from build123d import *

# Parameters (mm, degrees)
F1_DEPTH = 70
F2_R     = 50
F3_T     = -5


with BuildPart() as f1:
    # F0 (on Front) → F1 (new body)
    with BuildSketch(Plane.XZ):
        with BuildLine():
            Line((195.61244, 127.258498), (-44.38756, 127.258498))
            ThreePointArc((-44.38756, 127.258498), (-83.278433, 111.149371), (-99.38756, 72.258498))
            ThreePointArc((-99.38756, 72.258498), (-83.278433, 33.367625), (-44.38756, 17.258498))
            Line((-44.38756, 17.258498), (195.61244, 17.258498))
            ThreePointArc((195.61244, 17.258498), (234.503313, 33.367625), (250.61244, 72.258498))
            ThreePointArc((250.61244, 72.258498), (234.503313, 111.149371), (195.61244, 127.258498))
        make_face()
    extrude(amount=F1_DEPTH)

    # F2
    f2_edges = [f1.edges().sort_by_distance(p)[0] for p in [
        (75.61244, -70, 127.258498),
        (-99.38756, -70, 72.258498),
        (75.61244, -70, 17.258498),
        (250.61244, -70, 72.258498),
    ]]
    fillet(f2_edges, radius=F2_R)

    # F3
    f3_openings = [f1.faces().sort_by_distance(p)[0] for p in [
        (75.61244, 0, 72.258498),
    ]]
    offset(amount=F3_T, openings=f3_openings)


solid = f1.part
Geometry check sheet. Reference: the model listing, model coordinates, mm. A direction names the side the tool comes from. Give positions to 0.01 mm unless a question says otherwise; leave off trailing zeros. Loops run counter-clockwise (first coordinate to the right, second up) from the corner with the lowest first, then second, coordinate; pieces in that order, holes last. Notation, with made-up numbers: M -23,38.5 L -1,38.5 A23 cw -1,63.5 Z; hole C 82.25,-13.75 d5. An arc over 180 degrees is marked long. Answer as a JSON object with one key per item and string values. Group by question number.
Item 1: Access from +Z, -Z, +X, -X, +Y, -Y to the whole of each face (thin tool, end or side, straight path). Record for faces 3 (the cylindrical face through (77.29, -51.47, 35.09)), 4 (the flat face through (74, -10, 17.258)).
Item 2: Sectioned sample at A-A on y = -15. Record the boundary of the cut face in (x, z).
Item 3: Sectioned sample at B-B on x = 176. Record the boundary of the cut face in (y, z), plus the area to 3 significant figures.
Item 4: Material ranges on L1, parallel to Z at x = 114, y = -19.5; L2, parallel to X at y = -28, z = 91; L3, parallel to X at y = -3, z = 70.5, recorded low to high.
Item 5: Mould release check, pull along X, two halves, no side actions. Record for faces 1 (the flat face through (74, -10, 22.258)), 2 (the cylindrical face through (73.932, -54.964, 113)): pulls with the +X half, pulls with the -X half, needs draft (parallel to the pull), parting line crosses it, or undercut.
Item 6: Gauge pin test, flat ends, axial feed: pin 1 (12 mm diameter, centred on x = 127.5, z = 39, fed in from +Y); pin 2 (8 mm diameter, centred on y = -31, z = 45.5, fed in from +X); pin 3 (3 mm diameter, centred on y = -22, z = 49, fed in from +X) (3 decimals). Record the tip position at first contact, or that the pin passes through.
Findings below:
{
 "1": {"face 3": "+Y", "face 4": "-Z, +X, -X, +Y, -Y"},
 "2": {"outline": "M -44.39,17.26 L 195.61,17.26 A55 ccw 195.61,127.26 L -44.39,127.26 A55 ccw Z; hole M -44.39,22.26 L 195.61,22.26 A50 ccw 195.61,122.26 L -44.39,122.26 A50 ccw Z"},
 "3": {"outline": "M -70,67.26 A50 ccw -20,17.26 L 0,17.26 L 0,22.26 L -20,22.26 A45 cw -65,67.26 L -65,77.26 A45 cw -20,122.26 L 0,122.26 L 0,127.26 L -20,127.26 A50 ccw -70,77.26 Z", "area": "996 mm2"},
 "4": {"L1": "17.26 to 22.26, 122.26 to 127.26", "L2": "-95.41 to -89.97, 241.19 to 246.64", "L3": "-99.36 to -94.36, 245.58 to 250.58"},
 "5": {"face 1": "undercut", "face 2": "needs draft"},
 "6": {"pin 1": "y = -49.18", "pin 2": "x = 244.55", "pin 3": "x = 246.085"}
}
